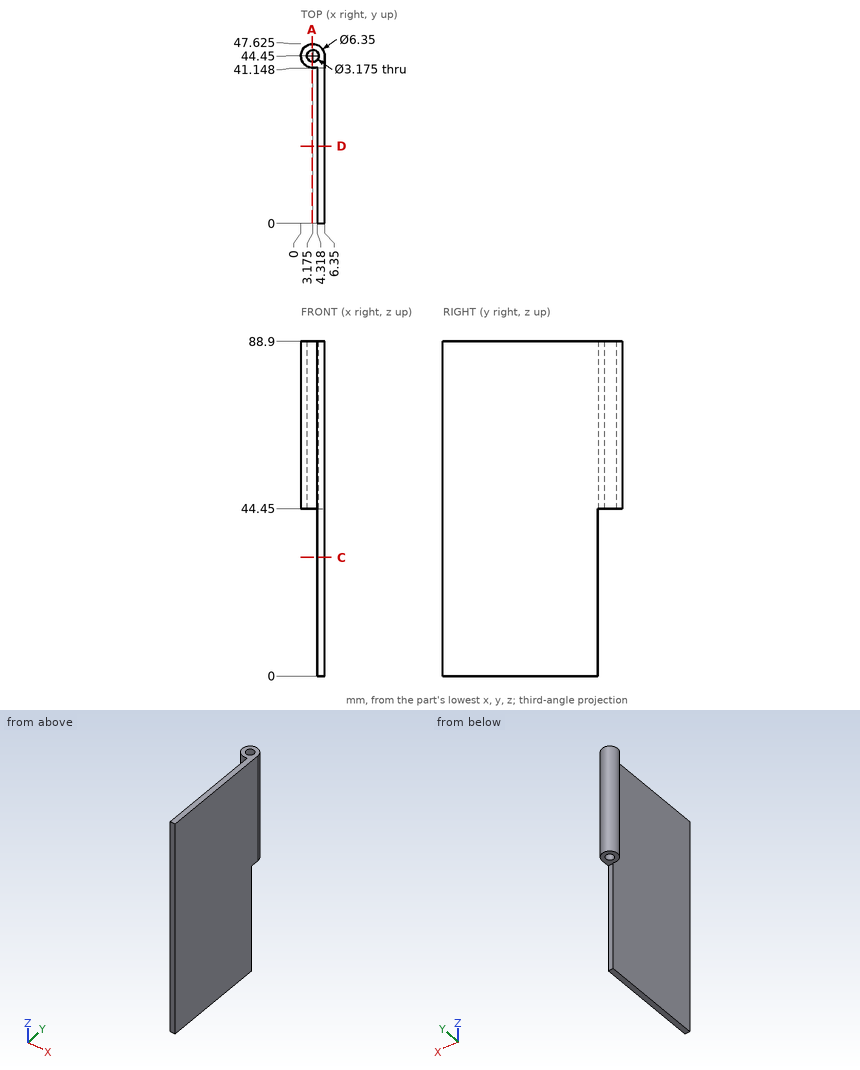
The drawing under review shows one solid part. Ordinate dimensions are in mm from its lowest x, y, z. Round coordinates to 2 decimals unless told otherwise and drop trailing zeros. Write each loop counter-clockwise with the first axis right and the second up, starting at its lowest first coordinate (ties: lowest second). Pieces come first, ordered by that corner, then holes. Notation, with made-up numbers: M 62,60 L 81,60 A26 ccw 81,75 Z; hole C 88.25,-28 d9. An arc over 180 degrees is marked long. One line per item, written item: value. Start each with the question number.
(1) We need section C-C (z = 31.5). Give the boundary of the cut face in (x, y).
(2) Insertion check: pin 1 (3 mm diameter, centred on x = 4, y = 43.5, fed in from -Z); pin 2 (2 mm diameter, centred on x = 5.5, z = 15, fed in from +Y). Each pin has a flat end and moves straight along its axis. Give the tip position at first contact, or say it passes through.
(3) Wall thickness on line 1 (X direction, y = 44.45, z = 58); line 2 (Y direction, x = 6, z = 24.5); line 3 (Y direction, x = 4, z = 62): over which ranges is each line inside the solid? List them lowest first.
(4) We need section A-A (x = 3). Give the boundary of the cut face in (y, z).
(5) We need section D-D (y = 20.5). Give the boundary of the cut face in (x, z), and give its area (3 significant figures).
Result:
1. outline: M 4.32,0 L 6.35,0 L 6.35,41.15 L 4.32,41.15 Z
2. pin 1: z = 44.45
2. pin 2: y = 41.15
3. line 1: 0 to 1.59, 4.76 to 6.35
3. line 2: 0 to 41.15
3. line 3: 41.38 to 43.09, 45.81 to 47.52
4. outline: M 41.28,44.45 L 42.87,44.45 L 42.87,88.9 L 41.28,88.9 Z; M 46.03,44.45 L 47.62,44.45 L 47.62,88.9 L 46.03,88.9 Z
5. outline: M 4.32,0 L 6.35,0 L 6.35,88.9 L 4.32,88.9 Z
5. area: 181 mm²
